Design review of the part built by this model. Coordinates are the model's own, in mm. A direction names the side the tool comes from. Coordinates: 2 decimals unless noted, no trailing zeros. Order: outer loops, then holes, each group sorted by start corner. A loop starts at its lowest first (then second) coordinate and runs counter-clockwise, first axis right, second up. Notation, with made-up numbers: (3.5, 7.5) -> (41.5, 7.5) arc R24 cw to (41.5, 24.5) -> close; hole circle Ø9 at (7.25, -28.5). An arc over 180 degrees is marked (long way). Use a Markdown table: item, result. Add a question column.
Q1. The part is to be moulded in two halves that separate along Y. For faces 1 (the face through (-26, 8.6, 5)), 2 (the face through (-25, -9, 10)), say which applies: pulls with the +Y half, pulls with the -Y half, needs draft (parallel to the pull), parting line crosses it, or undercut.
Q2. Add section D-D (y = -2.5). State the section outline as (x, z) points.
Q3. Machinability: for faces 3 (the face through (-3, 6.6, 5)), 4 (the face through (-6.5, -8, 5)), 5 (the face through (-25, -9, 0)), which of the approach directions +Z, -Z, +X, -X, +Y, -Y give a long, thin tool a straight path to every point of the face, cutting with its end or side? Answer none if there is none.
Q4. Insertion check: pin 1 (6 mm diameter, centred on x = -14.5, y = 5.5, fed in from -Z); pin 2 (3 mm diameter, centred on y = 4, z = 7, fed in from +X). Each pin has a flat end and moves straight along its axis. Give the tip position at first contact, or say it passes through.
Q5. Wall thickness on probe 1 along Y at (x, z) = (-26, 3); probe 2 along Y at (x, z) = (-1.5, 2.5); probe 3 along X at (y, z) = (6.75, 0.5): over which ranges is each line inside the solid? List them lowest first.
Q6. Add section C-C (z = 1.75). State the section outline as (x, y) points.
Q7. Add section B-B (x = -2.5). State the section outline as (y, z) points, then the cut area to 3 significant figures.
Q8. Add section A-A (y = 8). State the section outline as (x, z) points, then the cut area to 3 significant figures.
from build123d import *

# Parameters (mm, degrees)
F0_W     = 6.5
F0_H     = 2
F1_DEPTH = 10


# Not quite as in the source:
# - ends of sketch curves that miss each other by under 0.0002 mm in the source are joined


with BuildPart() as f1:
    # F0 (on Top) → F1 (new body)
    with BuildSketch(Plane.XY):
        Polygon((-44.5, -8.6), (-44.5, 0), (-44.5, 8.6), (-6.5, 8.6), (0, 8.6), (0, 9.8000001162), (-5.5, 9.8000001162), (-45.7, 9.8), (-45.7, 0), (-45.7, -9.8), (-5.5, -9.8), (0, -9.8000001162), (0, -8.6), (0, -6.6), (-6.5, -6.6), (-6.5, -8.6), align=None)
        with Locations((-3.25, 7.6)):
            Rectangle(F0_W, F0_H)
    extrude(amount=F1_DEPTH)


solid = f1.part
Established:
| question | item | result |
|---|---|---|
| 1 | face 1 | undercut |
| 1 | face 2 | needs draft |
| 2 | outline | (-45.7, 0) -> (-44.5, 0) -> (-44.5, 10) -> (-45.7, 10) -> close |
| 3 | face 3 | +Z, -Z, +X |
| 3 | face 4 | +Z, -Z |
| 3 | face 5 | -Z, +X, -X, +Y, -Y |
| 4 | pin 1 | through |
| 4 | pin 2 | x = -44.5 |
| 5 | probe 1 | -9.8 to -8.6, 8.6 to 9.8 |
| 5 | probe 2 | -9.8 to -6.6, 6.6 to 9.8 |
| 5 | probe 3 | -45.7 to -44.5, -6.5 to 0 |
| 6 | outline | (-45.7, -9.8) -> (0, -9.8) -> (0, -6.6) -> (-6.5, -6.6) -> (-6.5, -8.6) -> (-44.5, -8.6) -> (-44.5, 8.6) -> (-6.5, 8.6) -> (-6.5, 6.6) -> (0, 6.6) -> (0, 9.8) -> (-45.7, 9.8) -> close |
| 7 | outline | (-9.8, 0) -> (-6.6, 0) -> (-6.6, 10) -> (-9.8, 10) -> close; (6.6, 0) -> (9.8, 0) -> (9.8, 10) -> (6.6, 10) -> close |
| 7 | area | 64.0 mm^2 |
| 8 | outline | (-45.7, 0) -> (-44.5, 0) -> (-44.5, 10) -> (-45.7, 10) -> close; (-6.5, 0) -> (0, 0) -> (0, 10) -> (-6.5, 10) -> close |
| 8 | area | 77.0 mm^2 |
